For this review, take the finished solid that the model builds, in its own axes (mm). A direction names the side the tool comes from. Round coordinates to 2 decimals unless told otherwise and drop trailing zeros. Order: outer loops, then holes, each group sorted by start corner. A loop starts at its lowest first (then second) coordinate and runs counter-clockwise, first axis right, second up. Notation, with made-up numbers: M -5,23 L 53,23 A23 ccw 53,43 Z; hole C 32.25,76.25 d9. An arc over 180 degrees is marked long. Put each result on its own line as item: value.
from build123d import *

# Parameters (mm, degrees)
CROQUIS1_W              = 20
CROQUIS1_H              = 30
CROQUIS1_R              = 1.65
SALIENTE_EXTRUIR1_DEPTH = 3
CORTAR_EXTRUIR1_REACH   = 5


with BuildPart() as part:
    # Croquis1 → Saliente-Extruir1 (new body)
    with BuildSketch(Plane.XY):
        Rectangle(CROQUIS1_W, CROQUIS1_H)
        with Locations((-7, 12)):
            Circle(CROQUIS1_R, mode=Mode.SUBTRACT)
        with Locations((7, 12)):
            Circle(CROQUIS1_R, mode=Mode.SUBTRACT)
        with Locations((7, -12)):
            Circle(CROQUIS1_R, mode=Mode.SUBTRACT)
        with Locations((-7, -12)):
            Circle(CROQUIS1_R, mode=Mode.SUBTRACT)
    extrude(amount=SALIENTE_EXTRUIR1_DEPTH)

    # Croquis2 → Cortar-Extruir1 (cut, up to next)
    with BuildSketch(Plane.XY.offset(3), mode=Mode.PRIVATE) as cortar_extruir1_sk1:
        with BuildLine():
            Line((-5, -4), (-5, 4))
            ThreePointArc((-5, 4), (0, 9), (5, 4))
            Line((5, 4), (5, -4))
            ThreePointArc((5, -4), (0, -9), (-5, -4))
        make_face()
    cortar_extruir1_tool1 = extrude(cortar_extruir1_sk1.sketch, amount=-CORTAR_EXTRUIR1_REACH, mode=Mode.PRIVATE) & part.part
    add(cortar_extruir1_tool1.solids().sort_by_distance((0, 0, 3))[0], mode=Mode.SUBTRACT)


solid = part.part
(1) Add section B-B on y = 12. Give the boundary of the cut face in (x, z), then the cut area to 3 significant figures.
A:
outline: M -10,0 L -8.65,0 L -8.65,3 L -10,3 Z; M -5.35,0 L 5.35,0 L 5.35,3 L -5.35,3 Z; M 8.65,0 L 10,0 L 10,3 L 8.65,3 Z
area: 40.2 mm2
(2) To check wall thickness, follow L1, parallel to Y at x = 7, z = 1.75; L2, parallel to X at y = 3.75, z = 0.5; L3, parallel to Y at x = 0.25, z = 0.85. State the ranges of each line that lie inside material, in increasing order.
A:
L1: y = -15 to -13.65, -10.35 to 10.35, 13.65 to 15
L2: x = -10 to -5, 5 to 10
L3: y = -15 to -8.99, 8.99 to 15
(3) Add section A-A on x = 0. Give the boundary of the cut face in (y, z).
A:
outline: M -15,0 L -9,0 L -9,3 L -15,3 Z; M 9,0 L 15,0 L 15,3 L 9,3 Z
(4) Add section C-C on z = 0.35. Give the boundary of the cut face in (x, y).
A:
outline: M -10,-15 L 10,-15 L 10,15 L -10,15 Z; hole C -7,-12 d3.3; hole C -7,12 d3.3; hole M -5,-4 A5 ccw 5,-4 L 5,4 A5 ccw -5,4 Z; hole C 7,-12 d3.3; hole C 7,12 d3.3
(5) Draft analysis for pull direction X (two halves, no side actions). For faces 1 (the face through (10, 0, 1)), 2 (the face through (-10, 0, 1)), 3 (the face through (-5, 0, 2)), state which applies: released by +X, released by -X, zero draft, split by the parting line, or undercut.
A:
face 1: released by +X
face 2: released by -X
face 3: undercut
(6) For faces 4 (the face through (0, -15, 1)), 5 (the face through (0, -9, 2)), list the 3-axis set-ups (+Z, -Z, +X, -X, +Y, -Y) from which the entire face can be reached by the end or side of a thin tool; tool diameter is ignored.
A:
face 4: +Z, -Z, +X, -X, -Y
face 5: +Z, -Z
(7) Add section D-D on x = -7. Give the boundary of the cut face in (y, z), then the cut area to 3 significant figures.
A:
outline: M -15,0 L -13.65,0 L -13.65,3 L -15,3 Z; M -10.35,0 L 10.35,0 L 10.35,3 L -10.35,3 Z; M 13.65,0 L 15,0 L 15,3 L 13.65,3 Z
area: 70.2 mm2
